from build123d import *

# Parameters (mm, degrees)
ESBO_O1_W                = 20
ESBO_O1_H                = 40
ESBO_O1_W_2              = 16
ESBO_O1_H_2              = 36
RESSALTO_EXTRUS_O1_DEPTH = 300
ESBO_O2_R                = 1.75
CORTE_EXTRUS_O1_DEPTH    = 2


with BuildPart() as part:
    # Esboço1 → Ressalto-extrusão1 (new body)
    with BuildSketch(Plane.XY):
        with Locations((10, 20)):
            Rectangle(ESBO_O1_W, ESBO_O1_H)
        with Locations((10, 20)):
            Rectangle(ESBO_O1_W_2, ESBO_O1_H_2, mode=Mode.SUBTRACT)
    extrude(amount=RESSALTO_EXTRUS_O1_DEPTH)

    # Esboço2 → Corte-extrusão1 (cut)
    with BuildSketch(Plane.ZY):
        with Locations((10, 30)):
            Circle(ESBO_O2_R)
        with Locations((10, 15)):
            Circle(ESBO_O2_R)
        with Locations((70, 15)):
            Circle(ESBO_O2_R)
        with Locations((55, 15)):
            Circle(ESBO_O2_R)
        with Locations(Location((230, 15, 0), (0, 0, 180))):
            Circle(ESBO_O2_R)
        with Locations(Location((245, 15, 0), (0, 0, 180))):
            Circle(ESBO_O2_R)
        with Locations(Location((290, 15, 0), (0, 0, 180))):
            Circle(ESBO_O2_R)
        with Locations(Location((290, 30, 0), (0, 0, 180))):
            Circle(ESBO_O2_R)
    extrude(amount=-CORTE_EXTRUS_O1_DEPTH, mode=Mode.SUBTRACT)


solid = part.part
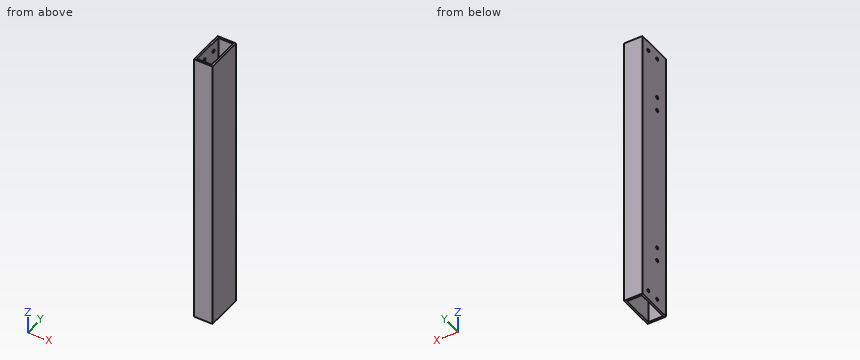
Source: CAD feature listing. Evaluate the final solid. Frame: model axes, mm. Round coordinates to 2 decimals unless told otherwise and drop trailing zeros. Loops run counter-clockwise (first coordinate to the right, second up) from the corner with the lowest first, then second, coordinate; pieces in that order, holes last.
Q1. Ray query, line 1 (Y direction, x = 1, z = 10); line 2 (X direction, y = 20, z = 255.5); line 3 (Y direction, x = 8, z = 107.5). Return the intervals inside material, ascending.
Q2. Section C-C, the plane z = 221. Return loops of the section in (x, y), plus the area to 3 significant figures.
Q3. First-contact query: P1, Ø6, axis at x = 12.5, y = 11.5, coming from the +Z side; P2, Ø3, axis at y = 15, z = 70, coming from the -X side. Flat tips, straight axial feed; report the tip coordinate or a pass-through.
Q4. Section B-B, the plane x = 7.75. Return loops of the section in (y, z).
Q5. Section A-A, the plane y = 5. Return loops of the section in (x, z).
Solutions:
1. line 1: y = 0 to 13.25, 16.75 to 28.25, 31.75 to 40
1. line 2: x = 0 to 2, 18 to 20
1. line 3: y = 0 to 2, 38 to 40
2. outline: (0, 0) - (20, 0) - (20, 40) - (0, 40) - close; hole (2, 2) - (18, 2) - (18, 38) - (2, 38) - close
2. area: 224 mm2
3. P1: passes through
3. P2: stops at x = 18
4. outline: (0, 0) - (2, 0) - (2, 300) - (0, 300) - close; (38, 0) - (40, 0) - (40, 300) - (38, 300) - close
5. outline: (0, 0) - (2, 0) - (2, 300) - (0, 300) - close; (18, 0) - (20, 0) - (20, 300) - (18, 300) - close
